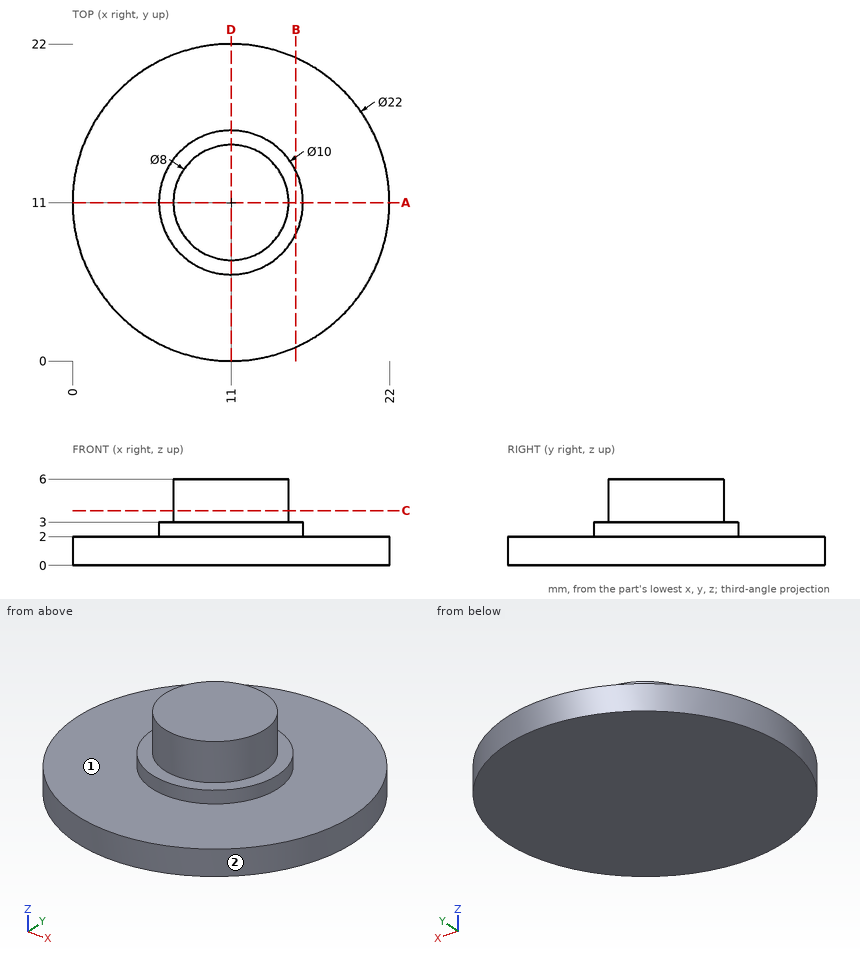
The figure shows three views and two pictorial views of one solid part (mm, origin at its lowest corner). Answer the questions. A direction names the side the tool comes from. Coordinates: 2 decimals unless noted, no trailing zeros. Write each loop counter-clockwise with the first axis right and the second up, starting at its lowest first coordinate (ties: lowest second). Pieces come first, ordered by that corner, then holes. Notation, with made-up numbers: (46, -25) -> (89, -25) arc R22 cw to (89, -12) -> close; hole circle Ø8 at (-34, 26.25). An arc over 180 degrees is marked (long way). Answer as a JSON object with one key per item and string values.
Q1. A flat-ended cylindrical pin translates along its axis: pin 1 Ø6 at (x, y) = (18.5, 11.5) entering from +Z. Find the tip coordinate at first contact, or state that the pin passes through.
The answers:
{"pin 1": "stops at z = 3"}
Q2. A tool of negligible diameter and unlimited length cuts with its end or side. For the marked faces 1 and 2, from which of +Z, -Z, +X, -X, +Y, -Y can it reach the whole face along a straight path? Write none if from no direction.
The answers:
{"face 1": "+Z", "face 2": "+Z, -Z"}
Q3. The part is cut by section B-B on x = 15.5. Give the vertices of the cut face in (y, z).
The answers:
{"outline": "(0.96, 0) -> (21.04, 0) -> (21.04, 2) -> (13.18, 2) -> (13.18, 3) -> (8.82, 3) -> (8.82, 2) -> (0.96, 2) -> close"}
Q4. The part is cut by section A-A on y = 11. Give the vertices of the cut face in (x, z), then the cut area to 3 significant figures.
The answers:
{"outline": "(0, 0) -> (22, 0) -> (22, 2) -> (16, 2) -> (16, 3) -> (15, 3) -> (15, 6) -> (7, 6) -> (7, 3) -> (6, 3) -> (6, 2) -> (0, 2) -> close", "area": "78.0 mm2"}
Q5. Consider line 1 (Z direction, x = 20.5, y = 9.5); line 2 (Z direction, x = 11.5, y = 6.25); line 3 (X direction, y = 15.5, z = 0.5). Determine where each line is inside the solid, lowest interval first. Write a range as [from, to].
The answers:
{"line 1": "z = [0, 2]", "line 2": "z = [0, 3]", "line 3": "x = [0.96, 21.04]"}
Q6. The part is cut by section C-C on z = 3.8. Give the vertices of the cut face in (x, y), then the cut area to 3 significant figures.
The answers:
{"outline": "circle Ø8 at (11, 11)", "area": "50.3 mm2"}
